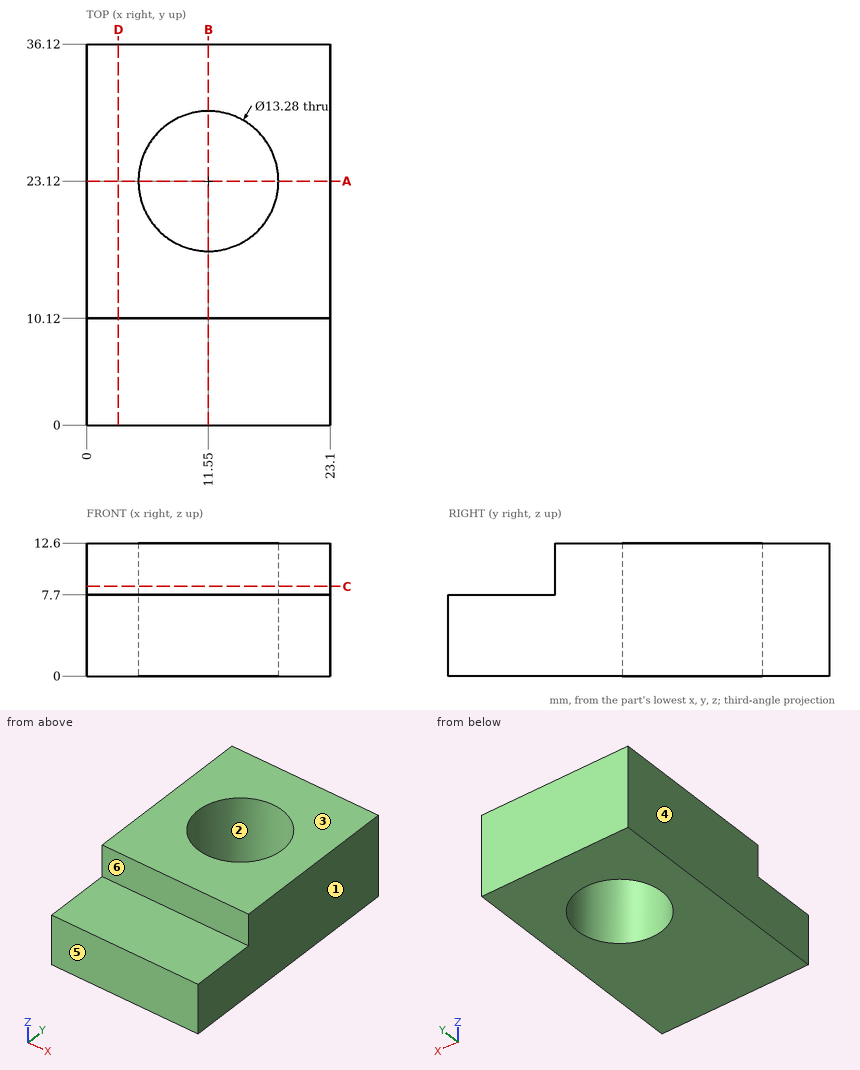
Print and shaded views of the part. All mm, measured from the part's lowest x, y and z. A direction names the side the tool comes from. Give positions to 0.01 mm unless a question says otherwise; leave off trailing zeros. Loops run counter-clockwise (first coordinate to the right, second up) from the corner with the lowest first, then second, coordinate; pieces in that order, holes last. Notation, with made-up numbers: (25.25, -7) - (46.25, -7) arc R6 cw to (46.25, 1) - close; hole circle Ø10 at (35.5, 33). An arc over 180 degrees is marked (long way). Use a Markdown table: item, result.
(1) Band-saw the part on B-B (x = 11.55). Give the cut face in (y, z).
Taken from the geometry:
| item | result |
|---|---|
| outline | (0, 0) - (16.48, 0) - (16.48, 12.6) - (10.12, 12.6) - (10.12, 7.7) - (0, 7.7) - close; (29.76, 0) - (36.12, 0) - (36.12, 12.6) - (29.76, 12.6) - close |
(2) Wall check: line 1 along Y through (x, z) = (11.55, 5); line 2 along Y through (x, z) = (11.75, 10.75); line 3 along Z through (x, y) = (8.25, 6). Give the ranges that are in metal, low to high.
Taken from the geometry:
| item | result |
|---|---|
| line 1 | 0 to 16.48, 29.76 to 36.12 |
| line 2 | 10.12 to 16.48, 29.76 to 36.12 |
| line 3 | 0 to 7.7 |
(3) Band-saw the part on C-C (z = 8.5). Give the cut face in (x, y).
Taken from the geometry:
| item | result |
|---|---|
| outline | (0, 10.12) - (23.1, 10.12) - (23.1, 36.12) - (0, 36.12) - close; hole circle Ø13.28 at (11.55, 23.12) |
(4) Band-saw the part on A-A (y = 23.12). Give the cut face in (x, z), and give its area (3 significant figures).
Taken from the geometry:
| item | result |
|---|---|
| outline | (0, 0) - (4.91, 0) - (4.91, 12.6) - (0, 12.6) - close; (18.19, 0) - (23.1, 0) - (23.1, 12.6) - (18.19, 12.6) - close |
| area | 124 mm2 |
(5) Pull direction X, two halves, no side cores. Call the marked faces 1, 2, 3 and 4: +X half, -X half, draft (parallel to the pull), parting line (faces both ways), or undercut.
Taken from the geometry:
| item | result |
|---|---|
| face 1 | +X half |
| face 2 | undercut |
| face 3 | draft |
| face 4 | -X half |
(6) Band-saw the part on D-D (x = 3). Give the cut face in (y, z), and give its area (3 significant figures).
Taken from the geometry:
| item | result |
|---|---|
| outline | (0, 0) - (36.12, 0) - (36.12, 12.6) - (10.12, 12.6) - (10.12, 7.7) - (0, 7.7) - close |
| area | 406 mm2 |
(7) Which spindle directions (+Z, -Z, +X, -X, +Y, -Y) get a long thin tool onto all of the face, cutting with end or side? Do the marked faces 5 and 6. Say none if no direction does.
Taken from the geometry:
| item | result |
|---|---|
| face 5 | +Z, -Z, +X, -X, -Y |
| face 6 | +Z, +X, -X, -Y |
(8) Drop flat-ended pins along their axis: pin 1 Ø2 at (y, z) = (7, 9) entering from -X; pin 2 Ø1.5 at (x, z) = (8, 11) entering from -Y. Give the stop position or say it passes through.
Taken from the geometry:
| item | result |
|---|---|
| pin 1 | through |
| pin 2 | y = 10.12 |
